For this review, take the finished solid that the model builds, in its own axes (mm). A direction names the side the tool comes from. Give positions to 0.01 mm unless a question says otherwise; leave off trailing zeros. Order: outer loops, then holes, each group sorted by start corner. A loop starts at its lowest first (then second) coordinate and runs counter-clockwise, first axis right, second up. Notation, with made-up numbers: (36.5, -5) - (95.5, -5) arc R23 ccw to (95.5, 27) - close; hole circle Ø9 at (-19.75, 54). An arc over 180 degrees is marked (long way). Use a Markdown table: item, result. Add a question column.
1) We need section B-B on z = 3.75. Write out the cut boundary in (x, y), then the cut area to 3 significant figures.
2) We need section A-A on y = 1.5. Write out the cut boundary in (x, z), then the cut area to 3 significant figures.
3) Wall thickness on L1, parallel to X at y = -2.85, z = 2.5; L2, parallel to X at y = 0.55, z = -4; L3, parallel to Z at x = 1.75, y = -3.5: over which ranges is each line inside the solid? List them lowest first.
4) We need section D-D on z = -6.25. Write out the cut boundary in (x, y).
5) Clearance check with flat-ended pins moving along their axes: P1, Ø2.5, axis at x = 2.5, z = -1.5, coming from the +Y side; P2, Ø1.6, axis at x = 0.5, z = -4, coming from the +Y side; P3, Ø2.5, axis at x = -1.5, z = -5.5, coming from the +Y side. State where each tip first meets the part, or that it passes through.
6) Machinability: for faces 1 (the face through (2, -2, 5)), 2 (the face through (3, 1, 5)), 3 (the face through (-0.1, 2.2, -5.7)), which of the approach directions +Z, -Z, +X, -X, +Y, -Y give a long, thin tool a straight path to every point of the face, cutting with its end or side? Answer none if there is none.
7) Mouldability with a two-part tool opening along Y and no side actions: class faces 4 (the face through (-1, 1, -3)), 5 (the face through (2, 0, 0)), 6 (the face through (0.1, 1.5, -2.5)) as released by +Y, released by -Y, zero draft, split by the parting line, or undercut.
8) We need section C-C on y = -1.75. Write out the cut boundary in (x, z), then the cut area to 3 significant figures.
```python
from build123d import *

# Parameters (mm, degrees)
BOSS_EXTRUDE1_DEPTH = 7.5
SKETCH2_R           = 0.5
SKETCH2_R_2         = 3
CUT_EXTRUDE1_DEPTH  = 15
CUT_EXTRUDE2_DEPTH  = 3
CUT_EXTRUDE3_DEPTH  = 2
CUT_EXTRUDE4_DEPTH  = 2
CUT_EXTRUDE5_DEPTH  = 3
SKETCH8_R           = 1
CUT_EXTRUDE6_DEPTH  = 2


with BuildPart() as part:
    # Sketch1 → Boss-Extrude1 (new body, symmetric)
    with BuildSketch(Plane.XY):
        Polygon((-5, 4), (-5, -4), (5, -4), (5, 4), (4, 4), (4, 3), (-4, 3), (-4, 4), align=None)
    extrude(amount=BOSS_EXTRUDE1_DEPTH, both=True)

    # Sketch2 → Cut-Extrude1 (cut)
    with BuildSketch(Plane(origin=(0, 4, 0), x_dir=(1, 0, 0), z_dir=(0, 1, 0))):
        with BuildLine():
            Line((-5, 7.5), (-5, 6.5))
            ThreePointArc((-5, 6.5), (-2.549509757, 7.247548784), (0, 7.5))
            Line((0, 7.5), (-5, 7.5))
        make_face()
        with BuildLine():
            Line((4, 7.5), (0, 7.5))
            ThreePointArc((0, 7.5), (2.02470746, 7.341361287), (4, 6.869316877))
            Line((4, 6.869316877), (4, 7.5))
        make_face()
        with BuildLine():
            Line((5, 7.5), (4, 7.5))
            Line((4, 7.5), (4, 6.869316877))
            ThreePointArc((4, 6.869316877), (4.503787155, 6.694912926), (5, 6.5))
            Line((5, 6.5), (5, 7.5))
        make_face()
        with Locations((0, 4)):
            Circle(SKETCH2_R)
        with BuildLine():
            Line((-5, -7.5), (0, -7.5))
            ThreePointArc((0, -7.5), (-2.915475947, -6.692459912), (-5, -4.5))
            Line((-5, -4.5), (-5, -7.5))
        make_face()
        with BuildLine():
            ThreePointArc((5, -4.5), (4.550135794, -5.210813958), (4, -5.847198193))
            Line((4, -5.847198193), (4, -7.5))
            Line((4, -7.5), (5, -7.5))
            Line((5, -7.5), (5, -4.5))
        make_face()
        with BuildLine():
            Line((4, -7.5), (4, -5.847198193))
            ThreePointArc((4, -5.847198193), (2.164009809, -7.070524628), (0, -7.5))
            Line((0, -7.5), (4, -7.5))
        make_face()
        with Locations((0, -2.5)):
            Circle(SKETCH2_R_2)
    extrude(amount=-CUT_EXTRUDE1_DEPTH, mode=Mode.SUBTRACT)

    # Sketch4 → Cut-Extrude2 (cut)
    with BuildSketch(Plane(origin=(0, 3, 0), x_dir=(1, 0, 0), z_dir=(0, 1, 0))):
        with BuildLine():
            Line((3, -2.5), (3, -9.188092465))
            ThreePointArc((3, -9.188092465), (0, -12.188092465), (-3, -9.188092465))
            Line((-3, -9.188092465), (-3, -2.5))
            ThreePointArc((-3, -2.5), (0, 0.5), (3, -2.5))
        make_face()
    extrude(amount=-CUT_EXTRUDE2_DEPTH, mode=Mode.SUBTRACT)

    # Sketch5 → Cut-Extrude3 (cut)
    with BuildSketch(Plane(origin=(0, 0, 0), x_dir=(1, 0, 0), z_dir=(0, 1, 0))):
        with BuildLine():
            Line((4, -2.5), (4, -8.475889446))
            ThreePointArc((4, -8.475889446), (0, -12.475889446), (-4, -8.475889446))
            Line((-4, -8.475889446), (-4, -2.5))
            ThreePointArc((-4, -2.5), (0, 1.5), (4, -2.5))
        make_face()
    extrude(amount=-CUT_EXTRUDE3_DEPTH, mode=Mode.SUBTRACT)

    # Sketch6 → Cut-Extrude4 (cut)
    with BuildSketch(Plane(origin=(0, 4, 0), x_dir=(1, 0, 0), z_dir=(0, 1, 0))):
        with BuildLine():
            Line((5, -2.5), (5, -8.536359525))
            ThreePointArc((5, -8.536359525), (0, -13.536359525), (-5, -8.536359525))
            Line((-5, -8.536359525), (-5, -2.5))
            ThreePointArc((-5, -2.5), (0, 2.5), (5, -2.5))
        make_face()
    extrude(amount=-CUT_EXTRUDE4_DEPTH, mode=Mode.SUBTRACT)

    # Sketch7 → Cut-Extrude5 (cut)
    with BuildSketch(Plane(origin=(0, 4, 0), x_dir=(1, 0, 0), z_dir=(0, 1, 0))):
        with BuildLine():
            Line((-5, -2.5), (-5, 4))
            ThreePointArc((-5, 4), (0, 5.700609733), (5, 4))
            Line((5, 4), (5, -2.5))
            ThreePointArc((5, -2.5), (0, 2.5), (-5, -2.5))
        make_face()
    extrude(amount=-CUT_EXTRUDE5_DEPTH, mode=Mode.SUBTRACT)

    # Sketch8 → Cut-Extrude6 (cut)
    with BuildSketch(Plane(origin=(0, 1, 0), x_dir=(1, 0, 0), z_dir=(0, 1, 0))):
        with Locations((0, 4)):
            Circle(SKETCH8_R)
    extrude(amount=-CUT_EXTRUDE6_DEPTH, mode=Mode.SUBTRACT)


solid = part.part
```
Checked values:
| question | item | result |
|---|---|---|
| 1 | outline | (-5, -4) - (-2.73, -4) - (-2.73, -2) - (-4, -2) - (-4, 0) - (-3, 0) - (-3, 2) - (-5, 2) - close; (2.73, -4) - (5, -4) - (5, 2) - (3, 2) - (3, 0) - (4, 0) - (4, -2) - (2.73, -2) - close |
| 1 | area | 21.1 mm² |
| 2 | outline | (-5, -6.5) arc R13 ccw to (5, -6.5) - (5, -4) arc R8.2 cw to (-5, -4) - close; (-5, 2.5) arc R5 ccw to (5, 2.5) - (5, 4.5) arc R5.67 ccw to (3, 6.64) - (3, 2.5) arc R3 cw to (-3, 2.5) - (-3, 6.64) arc R5.67 ccw to (-5, 4.5) - close |
| 2 | area | 58.3 mm² |
| 3 | L1 | -5 to -3, 3 to 5 |
| 3 | L2 | -5 to -1, 1 to 5 |
| 3 | L3 | -7.38 to 0.06, 4.94 to 7.22 |
| 4 | outline | (-5, -4) - (5, -4) - (5, 4) - (4, 4) - (4, 3) - (-4, 3) - (-4, 4) - (-5, 4) - close |
| 5 | P1 | y = 2 |
| 5 | P2 | y = 1 |
| 5 | P3 | y = 3 |
| 6 | face 1 | +Z |
| 6 | face 2 | +Z, +Y |
| 6 | face 3 | +Y |
| 7 | face 4 | released by +Y |
| 7 | face 5 | undercut |
| 7 | face 6 | zero draft |
| 8 | outline | (-5, -6.5) arc R13 ccw to (5, -6.5) - (5, 4.5) arc R5.67 ccw to (4, 5.85) - (4, 2.5) arc R4 cw to (-4, 2.5) - (-4, 5.85) arc R5.67 ccw to (-5, 4.5) - close; hole circle Ø1 at (0, -4) |
| 8 | area | 76.3 mm² |
